Geometry check sheet. Reference: the model listing, model coordinates, mm. Face numbers are marked on the shaded views. Coordinates: 2 decimals unless noted, no trailing zeros. Order: outer loops, then holes, each group sorted by start corner. A loop starts at its lowest first (then second) coordinate and runs counter-clockwise, first axis right, second up. Notation, with made-up numbers: (51, -29.5) - (88, -29.5) arc R15 ccw to (88, -22.5) - close; hole circle Ø9 at (24, -4). An arc over 180 degrees is marked (long way). Put each result on its own line as item: value.
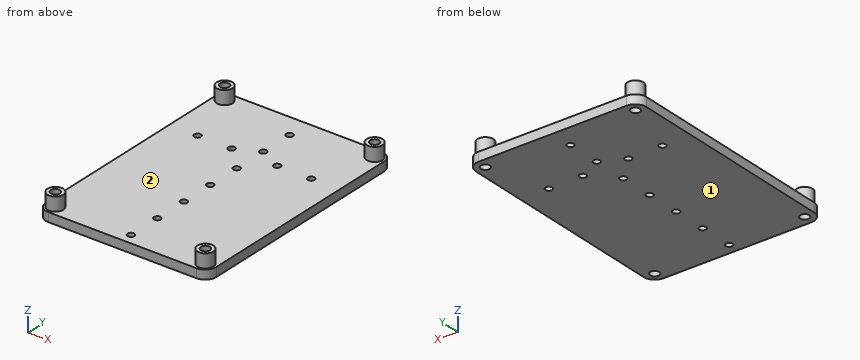
from build123d import *

# Parameters (mm, degrees)
SKETCH1_W           = 75
SKETCH1_H           = 105
SKETCH1_R           = 1.5
SKETCH1_R_2         = 2
BOSS_EXTRUDE1_DEPTH = 4
SKETCH2_R           = 3.5
SKETCH2_R_2         = 2
BOSS_EXTRUDE2_DEPTH = 6
FILLET1_R           = 5


with BuildPart() as part:
    # Sketch1 → Boss-Extrude1 (new body)
    with BuildSketch(Plane(origin=(0, 0, 116.694714263), x_dir=(-1, 0, 0), z_dir=(0, 0, -1))):
        with Locations((-134.526557277, 112.311918208)):
            Rectangle(SKETCH1_W, SKETCH1_H)
        with Locations((-134.526557277, 154.637085275)):
            Circle(SKETCH1_R, mode=Mode.SUBTRACT)
        with Locations((-134.526557277, 139.637085275)):
            Circle(SKETCH1_R, mode=Mode.SUBTRACT)
        with Locations((-144.526557277, 134.637085275)):
            Circle(SKETCH1_R, mode=Mode.SUBTRACT)
        with Locations((-159.526557277, 134.637085275)):
            Circle(SKETCH1_R, mode=Mode.SUBTRACT)
        with Locations((-124.526557277, 134.637085275)):
            Circle(SKETCH1_R, mode=Mode.SUBTRACT)
        with Locations((-109.526557277, 134.637085275)):
            Circle(SKETCH1_R, mode=Mode.SUBTRACT)
        with Locations((-134.526557277, 124.637085275)):
            Circle(SKETCH1_R, mode=Mode.SUBTRACT)
        with Locations((-134.526557277, 109.637085275)):
            Circle(SKETCH1_R, mode=Mode.SUBTRACT)
        with Locations((-134.526557277, 94.637085275)):
            Circle(SKETCH1_R, mode=Mode.SUBTRACT)
        with Locations((-134.526557277, 79.637085275)):
            Circle(SKETCH1_R, mode=Mode.SUBTRACT)
        with Locations((-134.526557277, 64.637085275)):
            Circle(SKETCH1_R, mode=Mode.SUBTRACT)
        with Locations((-167.526557277, 64.311918208)):
            Circle(SKETCH1_R_2, mode=Mode.SUBTRACT)
        with Locations((-101.526557277, 64.311918208)):
            Circle(SKETCH1_R_2, mode=Mode.SUBTRACT)
        with Locations((-101.526557277, 160.311918208)):
            Circle(SKETCH1_R_2, mode=Mode.SUBTRACT)
        with Locations((-167.526557277, 160.311918208)):
            Circle(SKETCH1_R_2, mode=Mode.SUBTRACT)
    extrude(amount=BOSS_EXTRUDE1_DEPTH)

    # Sketch2 → Boss-Extrude2 (add)
    with BuildSketch(Plane.XY.offset(116.694714263)):
        with Locations((101.526557277, 160.311918208)):
            Circle(SKETCH2_R)
        with Locations((101.526557277, 160.311918208)):
            Circle(SKETCH2_R_2, mode=Mode.SUBTRACT)
        with Locations((167.526557277, 160.311918208)):
            Circle(SKETCH2_R)
        with Locations((167.526557277, 160.311918208)):
            Circle(SKETCH2_R_2, mode=Mode.SUBTRACT)
        with Locations((101.526557277, 64.311918208)):
            Circle(SKETCH2_R)
        with Locations((101.526557277, 64.311918208)):
            Circle(SKETCH2_R_2, mode=Mode.SUBTRACT)
        with Locations((167.526557277, 64.311918208)):
            Circle(SKETCH2_R)
        with Locations((167.526557277, 64.311918208)):
            Circle(SKETCH2_R_2, mode=Mode.SUBTRACT)
    extrude(amount=BOSS_EXTRUDE2_DEPTH)

    # Fillet1
    fillet1_edges = [part.edges().sort_by_distance(p)[0] for p in [
        (172.026557277, 164.811918208, 114.694714263),
        (97.026557277, 164.811918208, 114.694714263),
        (97.026557277, 59.811918208, 114.694714263),
        (172.026557277, 59.811918208, 114.694714263),
    ]]
    fillet(fillet1_edges, radius=FILLET1_R)


solid = part.part
Q1. Section check B-B on y = 132. Record the boundary of the cut face in (x, z).
Answer block:
outline: (97.03, 112.69) - (172.03, 112.69) - (172.03, 116.69) - (97.03, 116.69) - close
Q2. Thickness scan on L1, parallel to Z at x = 106.5, y = 140; L2, parallel to X at y = 94.5, z = 115.75; L3, parallel to Y at x = 108.5, z = 114.5. Record the ranges inside material, lowest first. Write a range as [from, to].
Answer block:
L1: z = [112.69, 116.69]
L2: x = [97.03, 133.03], [136.02, 172.03]
L3: y = [59.81, 133.54], [135.73, 164.81]
Q3. Section check C-C on x = 128. Record the boundary of the cut face in (y, z), then the cut area to 3 significant figures.
Answer block:
outline: (59.81, 112.69) - (164.81, 112.69) - (164.81, 116.69) - (59.81, 116.69) - close
area: 420 mm^2
Q4. Draft check along X on the marked faces 1 and 2. Enter one of: pulls with the +X half, pulls with the -X half, needs draft (parallel to the pull), parting line crosses it, or undercut.
Answer block:
face 1: needs draft
face 2: undercut
Q5. Depth check by flat-ended pin: pin 1 Ø5 at (x, y) = (167.53, 160.31) entering from -Z; pin 2 Ø3.5 at (x, y) = (101.53, 64.31) entering from +Z; pin 3 Ø3.5 at (x, y) = (134.53, 124.64) entering from +Z. Enter the tip coordinate at first touch or a pass-through.
Answer block:
pin 1: stops at z = 112.69
pin 2: passes through
pin 3: stops at z = 116.69
Q6. Section check A-A on z = 119. Record the boundary of the cut face in (x, y), then the cut area to 3 significant figures.
Answer block:
outline: circle Ø7 at (101.53, 64.31); circle Ø7 at (101.53, 160.31); circle Ø7 at (167.53, 64.31); circle Ø7 at (167.53, 160.31); hole circle Ø4 at (101.53, 64.31); hole circle Ø4 at (101.53, 160.31); hole circle Ø4 at (167.53, 64.31); hole circle Ø4 at (167.53, 160.31)
area: 104 mm^2
